The model under review builds one solid part; all positions refer to its coordinate system, in mm. Coordinates: 2 decimals unless noted, no trailing zeros. Order: outer loops, then holes, each group sorted by start corner. A loop starts at its lowest first (then second) coordinate and runs counter-clockwise, first axis right, second up. Notation, with made-up numbers: M -5,40.25 L 5,40.25 A16 cw 5,52.25 Z; hole C -11,15 d1. An arc over 180 degrees is marked long. Write each question's results on one line, items separated by ' | '.
from build123d import *

# Parameters (mm, degrees)
F0_R      = 20.8202658932
F1_DEPTH  = 76.2
F1_FACE_R = 20.8202658932
F3_R      = 22.86


# Not quite as in the source:
# - an extrude whose draft closes it to a point is written as a loft to that point


with BuildPart() as f1:
    # F0 (on Front) → F1 (new body)
    with BuildSketch(Plane.XZ):
        Circle(F0_R)
    extrude(amount=F1_DEPTH)

    # F1_face (on face) → F2 section 0
    with BuildSketch(Plane.XZ.offset(76.2), mode=Mode.PRIVATE) as f2_s0:
        Circle(F1_FACE_R)
    loft([f2_s0.sketch, Vertex(0, -101.0126266769, 0)], ruled=True)

    # F3
    f3_edges = [f1.edges().sort_by_distance(p)[0] for p in [
        (-20.820266, -76.2, 0),
    ]]
    fillet(f3_edges, radius=F3_R)


solid = f1.part
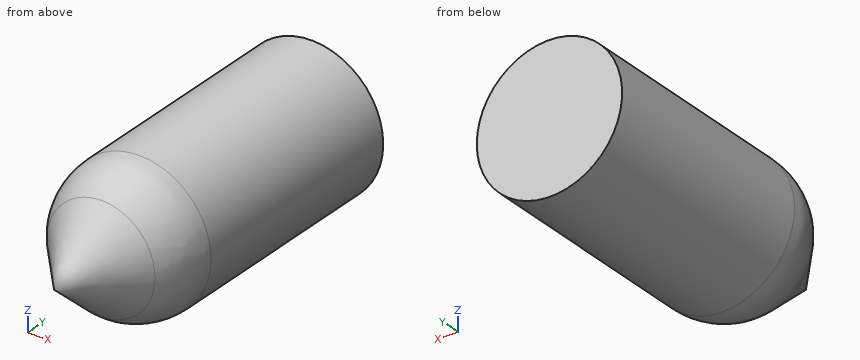
1) Take a section at A-A on y = -15. State the section outline as (x, z) points, plus the area to 3 significant figures.
Solutions:
outline: C 0,0 d41.64 | area: 1,360 mm2
2) To check wall thickness, follow line 1 along Z through (x, y) = (-0.5, -32); line 2 along Z through (x, y) = (-11.5, -22); line 3 along Y through (x, z) = (13, 1.5). State the ranges of each line that lie inside material, in increasing order.
Solutions:
line 1: -20.81 to 20.81 | line 2: -17.36 to 17.36 | line 3: -85.42 to 0
3) For pin 1 (6 mm diameter, centred on x = -14.5, z = -12.5, fed in from -Y); pin 2 (2 mm diameter, centred on x = 10.5, z = -5, fed in from -Y); pin 3 (8 mm diameter, centred on y = -36, z = 5.5, fed in from +X), all flat-tipped, find the tip position at first contact; note any pin that passes through.
Solutions:
pin 1: y = -81.73 | pin 2: y = -88.34 | pin 3: x = 20.77
